CAD build for the part. Positions are in the model's coordinates, mm. Give positions to 0.01 mm unless a question says otherwise; leave off trailing zeros. Write each loop counter-clockwise with the first axis right and the second up, starting at its lowest first coordinate (ties: lowest second). Pieces come first, ordered by that corner, then holes. Notation, with made-up numbers: (1, 89) -> (30, 89) arc R26 ccw to (30, 112) -> close; hole circle Ø5 at (18.5, 24). An arc over 180 degrees is marked (long way). Answer as a JSON object with one key per item and string values.
```python
from build123d import *

# Parameters (mm, degrees)
EXTRUDE_1_DEPTH = 11
FILLET_1_R      = 0.6


with BuildPart() as part:
    # Эскиз1 → Бобышка-Вытянуть1 (new body)
    with BuildSketch(Plane(origin=(0, 0, 0), x_dir=(1, 0, 0), z_dir=(0, 1, 0))):
        with BuildLine():
            Line((-9, 0), (-9, 92))
            ThreePointArc((-9, 92), (0, 101), (9, 92))
            Line((9, 92), (9, 0))
            ThreePointArc((9, 0), (0, -9), (-9, 0))
        make_face()
    extrude(amount=EXTRUDE_1_DEPTH)

    # Скругление1
    fillet_1_edges = [part.edges().sort_by_distance(p)[0] for p in [
        (0, 11, -101),
        (-9, 11, -46),
        (0, 11, 9),
        (-9, 0, -46),
        (0, 0, -101),
        (9, 0, -46),
        (0, 0, 9),
        (9, 11, -46),
    ]]
    fillet(fillet_1_edges, radius=FILLET_1_R)


solid = part.part
```
1) Wall check: probe 1 along X at (y, z) = (6.75, -92.5); probe 2 along Y at (x, z) = (-8.25, 2.5); probe 3 along Z at (x, y) = (-5.25, 10). Give the ranges that are in metal, low to high.
Model answer:
{"probe 1": "x = -8.99 to 8.99", "probe 2": "y = 0.04 to 10.96", "probe 3": "z = -99.31 to 7.31"}
2) Slice it at A-A (y = 8.5). List the corners of the cut face in (x, z).
Model answer:
{"outline": "(-9, -92) arc R9 ccw to (9, -92) -> (9, 0) arc R9 ccw to (-9, 0) -> close"}
3) Pin check, flat tip, straight feed: pin 1 (5 mm diameter, centred on x = -3.5, y = 3, fed in from +Z). Stop position of the tip, or through.
Model answer:
{"pin 1": "stops at z = 8.94"}
